Can you work these out from the model? Positions are in its coordinate system, mm. A direction names the side the tool comes from. Give positions to 0.01 mm unless a question says otherwise; leave off trailing zeros. One line per question, with ' | ' between items.
```python
from build123d import *

# Parameters (mm, degrees)
BOSS_EXTRUDE1_DEPTH         = 3.75
BOLT_HOLE_REACH             = 26.729
SKETCH2_R                   = 1.6
BOLT_HOLE_DIRECTION_2_REACH = 26.729
BOSS_EXTRUDE2_START         = 5
BOSS_EXTRUDE2_DEPTH         = 5
CUT_EXTRUDE2_START          = 11
SKETCH4_R                   = 2.85
CUT_EXTRUDE2_DEPTH          = 3
SKETCH7_RX                  = 10
SKETCH7_RY                  = 5
SKETCH11_W                  = 7.251223943
SKETCH11_H                  = 3.177760732
CUT_EXTRUDE3_DEPTH          = 20
CUT_EXTRUDE7_START          = -11
CUT_EXTRUDE7_DEPTH          = 10
CUT_EXTRUDE8_START          = -1.25
CUT_EXTRUDE8_DEPTH          = 1.828931


with BuildPart() as part:
    # Sketch1 → Boss-Extrude1 (new, symmetric)
    with BuildSketch(Plane.XY):
        with BuildLine():
            Line((-12.1, 0), (-14.051700625, -20))
            Line((-14.051700625, -20), (-10.051700625, -20))
            Line((-10.051700625, -20), (-8.425, -3.439385846))
            ThreePointArc((-8.425, -3.439385846), (0, 9.1), (8.425, -3.439385846))
            Line((8.425, -3.439385846), (10.051700625, -20))
            Line((10.051700625, -20), (14.051700625, -20))
            Line((14.051700625, -20), (12.1, 0))
            ThreePointArc((12.1, 0), (0, 12.1), (-12.1, 0))
        make_face()
    extrude(amount=BOSS_EXTRUDE1_DEPTH, both=True)

    # Bolt Hole: up to this plane
    bolt_hole_end = Plane(origin=(14.051700625, -20, 3.75), z_dir=(-0.995272319868323, -0.09712368044883128, 0))
    # Sketch2 → Bolt Hole (cut, up to the surface)
    with BuildSketch(Plane(origin=(0, 0, 0), x_dir=(0, 0, -1), z_dir=(1, 0, 0)), mode=Mode.PRIVATE) as bolt_hole_sk1:
        with Locations(Location((0, -10, 0), (0, 0, 90))):
            Circle(SKETCH2_R)
    bolt_hole_tool1 = split(extrude(bolt_hole_sk1.sketch, amount=BOLT_HOLE_REACH, mode=Mode.PRIVATE), bisect_by=bolt_hole_end, keep=Keep.BOTH, mode=Mode.PRIVATE)
    add(bolt_hole_tool1.solids().sort_by_distance((0, -10, 0))[0], mode=Mode.SUBTRACT)

    # Bolt Hole direction 2: up to this plane
    bolt_hole_direction_2_end = Plane(origin=(-12.1, 0, 3.75), z_dir=(0.995272319868323, -0.09712368044883138, 0))
    # Sketch2 → Bolt Hole direction 2 (cut, up to the surface)
    with BuildSketch(Plane(origin=(0, 0, 0), x_dir=(0, 0, -1), z_dir=(1, 0, 0)), mode=Mode.PRIVATE) as bolt_hole_direction_2_sk1:
        with Locations(Location((0, -10, 0), (0, 0, 90))):
            Circle(SKETCH2_R)
    bolt_hole_direction_2_tool1 = split(extrude(bolt_hole_direction_2_sk1.sketch, amount=-BOLT_HOLE_DIRECTION_2_REACH, mode=Mode.PRIVATE), bisect_by=bolt_hole_direction_2_end, keep=Keep.BOTH, mode=Mode.PRIVATE)
    add(bolt_hole_direction_2_tool1.solids().sort_by_distance((0, -10, 0))[0], mode=Mode.SUBTRACT)

    # Sketch3 → Boss-Extrude2 (add)
    with BuildSketch(Plane.XY.offset(3.75).offset(BOSS_EXTRUDE2_START)):
        with BuildLine():
            ThreePointArc((12.1, 0), (0, 12.1), (-12.1, 0))
            Line((-12.1, 0), (-6.05, 0))
            ThreePointArc((-6.05, 0), (0, 6.05), (6.05, 0))
            Line((6.05, 0), (12.1, 0))
        make_face()
        Polygon((-6.05, 0), (-12.1, 0), (-14.051700625, -20), (-8.001700625, -20), align=None)
        Polygon((14.051700625, -20), (12.1, 0), (6.05, 0), (8.001700625, -20), align=None)
    boss_extrude2 = extrude(amount=-BOSS_EXTRUDE2_DEPTH)

    # Sketch4 → Cut-Extrude2 (cut)
    with BuildSketch(Plane(origin=(0, 0, 0), x_dir=(0, 0, -1), z_dir=(1, 0, 0)).offset(CUT_EXTRUDE2_START)):
        with Locations(Location((0, -10, 0), (0, 0, 90))):
            Circle(SKETCH4_R)
    extrude(amount=CUT_EXTRUDE2_DEPTH, mode=Mode.SUBTRACT)

    # Sweep1: sweep along a path in Sketch8
    with BuildLine(Plane(origin=(0, 0, 0), x_dir=(0, 0, -1), z_dir=(1, 0, 0))) as sweep1_path:
        Line((20, 100), (0, 9.1))
    # Sketch7 → Sweep1 (sweep)
    with BuildSketch(Plane(origin=(0, 100, 0), x_dir=(1, 0, 0), z_dir=(0, 1, 0))):
        with Locations(Location((0, 20), (0, 0, -90))):
            Ellipse(SKETCH7_RX, SKETCH7_RY)
    sweep(path=sweep1_path.line)

    # Mirror2: Boss-Extrude2 across plane
    add(boss_extrude2.mirror(Plane.XY))

    # Sweep2: read off the stored shape, not the designer's step
    # Sweep2: loft between two sections, ruled curve by curve
    sweep2_from = [
        Edge.make_bspline([(-2.420614591, 9.1, -8.75), (-0.880223488, 9.1, -10.454545455), (0.880223488, 9.1, -10.454545455), (2.420614591, 9.1, -8.75)], [0, 0, 0, 0, 1, 1, 1, 1], 3, [1, 0.916666667, 0.916666667, 1]),
        Edge.make_line((2.420614591, 9.1, -8.75), (-2.420614591, 9.1, -8.75)),
    ]
    sweep2_to = [
        Edge.make_bspline([(-2.420614591, 3.41875, -7.5), (-0.880223488, 3.41875, -9.204545455), (0.880223488, 3.41875, -9.204545455), (2.420614591, 3.41875, -7.5)], [0, 0, 0, 0, 1, 1, 1, 1], 3, [1, 0.916666667, 0.916666667, 1]),
        Edge.make_line((2.420614591, 3.41875, -7.5), (-2.420614591, 3.41875, -7.5)),
    ]
    sweep2 = Solid(Shell([*[Face.make_surface_from_curves(sweep2_from[k], sweep2_to[k]) for k in range(2)], Face(Wire(sweep2_from)), Face(Wire(sweep2_to))]))
    add(sweep2)

    # Sketch11 → Cut-Extrude3 (cut)
    with BuildSketch(Plane(origin=(0, 0, 0), x_dir=(1, 0, 0), z_dir=(0, 1, 0))):
        with Locations((-0.008642554, -10.338880366)):
            Rectangle(SKETCH11_W, SKETCH11_H)
    extrude(amount=CUT_EXTRUDE3_DEPTH, mode=Mode.SUBTRACT)

    # Sketch14 → Cut-Extrude7 (cut)
    with BuildSketch(Plane(origin=(0, 0, 0), x_dir=(0, 0, -1), z_dir=(1, 0, 0)).offset(CUT_EXTRUDE7_START)):
        Polygon((-3.233161507, -10), (-1.616580754, -12.8), (1.616580754, -12.8), (3.233161507, -10), (1.616580754, -7.2), (-1.616580754, -7.2), align=None)
    extrude(amount=-CUT_EXTRUDE7_DEPTH, mode=Mode.SUBTRACT)

    # Sketch18 → Cut-Extrude8 (cut)
    with BuildSketch(Plane(origin=(0, 0, -8.75), x_dir=(-1, 0, 0), z_dir=(0, 0, -1)).offset(CUT_EXTRUDE8_START)):
        with BuildLine():
            Line((-6.05, 0), (6.05, 0))
            ThreePointArc((6.05, 0), (0, 6.05), (-6.05, 0))
        make_face()
    extrude(amount=CUT_EXTRUDE8_DEPTH, mode=Mode.SUBTRACT)


solid = part.part
```
(1) On a 3-axis mill with a long thin cutter (end or side, diameter ignored), from which of +Z, -Z, +X, -X, +Y, -Y can I reach the whole of each face in a straight line? I mean faces 1 (the face through (11.909, -12.847, 0.125)), 2 (the face through (7.012, -9.86, -6.285)), 3 (the face through (-9.25, -11.84, 0.05)), 4 (the face through (-0.249, 9.097, 0.053)), 5 (the face through (-12.158, -11.38, 2.436)). Say none if no direction works.
Answer below:
face 1: +X | face 2: +Z, -Z, -Y | face 3: -Y | face 4: none | face 5: -X
(2) If I drill on line 1 (Z direction, x = 10.4, y = -10); line 2 (Y direction, x = 10.2, z = 0); line 3 (Z direction, x = 11.7, y = -10), over which ranges is the centre line in solid material (lowest first)?
Answer below:
line 1: -8.75 to -1.6, 1.6 to 8.75 | line 2: -20 to -11.6, -8.4 to 6.51 | line 3: -8.75 to -2.85, 2.85 to 8.75
(3) Will these pins go through, and if not, where does the flat tip stop? pin 1 (2 mm diameter, centred on y = 65.5, z = 0, fed in from +X); pin 2 (6 mm diameter, centred on x = 8, y = 1.5, fed in from -Z); pin 3 (4.5 mm diameter, centred on y = -11, z = -1, fed in from +X); pin 4 (4.5 mm diameter, centred on y = -10, z = 0, fed in from +X).
Answer below:
pin 1: through | pin 2: z = -8.75 | pin 3: x = 13.39 | pin 4: x = 11
(4) Imagine slicing it at A-A (z = 0). Count the separate pieces of the cut face and the enclosed holes in it, and give its area (3 significant figures).
Answer below:
separate pieces: 3 | enclosed holes: 0 | area: 551 mm^2
(5) If we mould it in two halves opening along Y, with no side actions, what happens to faces 6 (the face through (9, -4, -8.75)), 7 (the face through (9.227, -11.604, 0.886)), 8 (the face through (-12.023, -8.62, -2.436))? For each: released by +Y, released by -Y, zero draft, split by the parting line, or undercut.
Answer below:
face 6: zero draft | face 7: released by -Y | face 8: undercut
